from build123d import *

# Parameters (mm, degrees)
SKETCH_1_W          = 15
SKETCH_1_H          = 15
SKETCH_1_W_2        = 13
SKETCH_1_H_2        = 13
EXTRUDE_1_DEPTH     = 240.3
SKETCH_2_R          = 1.45
CUT_EXTRUDE_1_DEPTH = 241.884495142
SKETCH_3_R          = 1.6
CUT_EXTRUDE_2_DEPTH = 241.884495142


with BuildPart() as part:
    # 草图1 → 凸台-拉伸1 (new body)
    with BuildSketch(Plane(origin=(0, 0, 0), x_dir=(0, 0, -1), z_dir=(1, 0, 0))):
        Rectangle(SKETCH_1_W, SKETCH_1_H)
        Rectangle(SKETCH_1_W_2, SKETCH_1_H_2, mode=Mode.SUBTRACT)
    extrude(amount=EXTRUDE_1_DEPTH)

    # 草图2 → 切除-拉伸1 (cut, through all)
    with BuildSketch(Plane(origin=(0, 7.5, 0), x_dir=(1, 0, 0), z_dir=(0, 1, 0))):
        with Locations(Location((233.3, 0, 0), (0, 0, 270))):
            Circle(SKETCH_2_R)
        with Locations(Location((226.3, 0, 0), (0, 0, 270))):
            Circle(SKETCH_2_R)
        with Locations(Location((14.99848481, 0, 0), (0, 0, 270))):
            Circle(SKETCH_2_R)
        with Locations(Location((4.99848481, 0, 0), (0, 0, 270))):
            Circle(SKETCH_2_R)
        with Locations(Location((29.99848481, 0, 0), (0, 0, 270))):
            Circle(SKETCH_2_R)
        with Locations(Location((39.99848481, 0, 0), (0, 0, 270))):
            Circle(SKETCH_2_R)
        with Locations(Location((49.99848481, 0, 0), (0, 0, 270))):
            Circle(SKETCH_2_R)
        with Locations(Location((104.99848481, 0, 0), (0, 0, 270))):
            Circle(SKETCH_2_R)
    extrude(amount=-CUT_EXTRUDE_1_DEPTH, mode=Mode.SUBTRACT)

    # 草图3 → 切除-拉伸2 (cut, through all)
    with BuildSketch(Plane.XY.offset(7.5)):
        with Locations((229.99848481, 0)):
            Circle(SKETCH_3_R)
        with Locations((189.99848481, 0)):
            Circle(SKETCH_3_R)
        with Locations((209.99848481, 0)):
            Circle(SKETCH_3_R)
    extrude(amount=-CUT_EXTRUDE_2_DEPTH, mode=Mode.SUBTRACT)


solid = part.part
Verification items for the finished model (mm, model axes). A direction names the side the tool comes from. Round coordinates to 2 decimals unless told otherwise and drop trailing zeros. Loops run counter-clockwise (first coordinate to the right, second up) from the corner with the lowest first, then second, coordinate; pieces in that order, holes last. Notation, with made-up numbers: (40.25, 49.5) - (77.25, 49.5) arc R19 ccw to (77.25, 70.5) - close; hole circle Ø3 at (51, 34). An arc over 180 degrees is marked (long way). Use one line per item in the form item = value.
1. Access from +Z, -Z, +X, -X, +Y, -Y to the whole of each face (thin tool, end or side, straight path). Record for faces 1 (the flat face through (118, 0, 6.5)), 2 (the flat face through (118, 0, 7.5)).
A:
face_1 = +X, -X
face_2 = +Z, +X, -X, +Y, -Y
2. Gauge pin test, flat end, axial feed: pin 1 Ø2.5 at (x, z) = (226.3, 0) entering from -Y. Record the tip position at first contact, or that the pin passes through.
A:
pin_1 = through
3. Draft check along Y on faces 3 (the flat face through (118, -7.5, 0)), 4 (the flat face through (118, 7.5, 0)), 5 (the flat face through (118, -6.5, 0)), 6 (the flat face through (240.3, 0, 7)). Enter one of: pulls with the +Y half, pulls with the -Y half, needs draft (parallel to the pull), parting line crosses it, or undercut.
A:
face_3 = pulls with the -Y half
face_4 = pulls with the +Y half
face_5 = undercut
face_6 = needs draft
4. Scan line: probe 1 along Z at (x, y) = (153.5, -1). Record every from-to range of solid material in increasing order.
A:
probe_1 = -7.5 to -6.5, 6.5 to 7.5
5. Section check A-A on x = 97.5. Record the cut outline in (y, z), and give its area (3 significant figures).
A:
outline = (-7.5, -7.5) - (7.5, -7.5) - (7.5, 7.5) - (-7.5, 7.5) - close; hole (-6.5, -6.5) - (6.5, -6.5) - (6.5, 6.5) - (-6.5, 6.5) - close
area = 56.0 mm²
